```python
from build123d import *

# Parameters (mm, degrees)
F0_W     = 30.6967236102
F0_H     = 108.7295114994
F2_T     = -5
F3_DEPTH = 25
F4_DEPTH = 172.6


with BuildPart() as f1:
    # F0 (on Front) → F1 (revolve)
    with BuildSketch(Plane.XZ):
        with Locations((-15.3483618051, 0)):
            Rectangle(F0_W, F0_H)
    revolve(axis=Axis((0, 0, -2.295082435), (0, 0, -1)))

    # F2
    f2_openings = [f1.faces().sort_by_distance(p)[0] for p in [
        (0, 0, 54.364756),
    ]]
    offset(amount=F2_T, openings=f2_openings)

    # F3 (add): a face of the model
    f3_faces = [f1.faces().sort_by_distance(p)[0] for p in [
        (0, 0, -49.3647557497),
    ]]
    extrude(f3_faces, amount=F3_DEPTH)

    # F4 (add): a face of the model
    f4_faces = [f1.faces().sort_by_distance(p)[0] for p in [
        (0, 0, -24.3647557497),
    ]]
    extrude(f4_faces, amount=F4_DEPTH)


solid = f1.part
```
Geometry: final body of the model. Coordinates: model frame, mm. A direction names the side the tool comes from. Round coordinates to 2 decimals unless told otherwise and drop trailing zeros. Order: outer loops, then holes, each group sorted by start corner. A loop starts at its lowest first (then second) coordinate and runs counter-clockwise, first axis right, second up. Notation, with made-up numbers: (46, 5.25) -> (69, 5.25) arc R13 ccw to (69, 20.25) -> close; hole circle Ø10 at (-31, 0). An arc over 180 degrees is marked (long way). Use one line per item in the form item = value. Start each with the question number.
1. Cut plane A-A (y = 0). Return the cut outline in (x, z), then the cut area to 3 significant figures.
2. Cut plane D-D (z = 119.5). Return the cut outline in (x, y), then the cut area to 3 significant figures.
3. Reachability of faces 1 (the face through (5.571, 25.086, 100.643)), 2 (the face through (0, 0, -54.365)) from +Z, -Z, +X, -X, +Y, -Y: full face, straight path, thin tool, end or side. Return the list, or none.
4. Cut plane B-B (x = 17). Return the cut outline in (y, z).
5. Pin query (flat end, axial travel): pin 1 Ø1.5 at (x, z) = (0, 123.5) entering from +Y; pin 2 Ø8 at (x, z) = (12.5, 106.5) entering from -Y; pin 3 Ø4 at (x, z) = (-1, -18) entering from -Y; pin 4 Ø8 at (y, z) = (2, 2.5) entering from -X. Return the tip coordinate at first contact, or that it passes through.
6. Line query: probe 1 along Z at (x, y) = (-24, 14.5); probe 2 along X at (y, z) = (1.5, 46.5); probe 3 along X at (y, z) = (0, 85). Output: solid intervals per line, ascending.
7. Cut plane C-C (z = 17.5). Return the cut outline in (x, y).
Solution:
q1.outline = (-30.7, -54.36) -> (30.7, -54.36) -> (30.7, 54.36) -> (25.7, 54.36) -> (25.7, 148.24) -> (-25.7, 148.24) -> (-25.7, 54.36) -> (-30.7, 54.36) -> close
q1.area = 11,500 mm^2
q2.outline = circle Ø51.39 at (0, 0)
q2.area = 2,070 mm^2
q3.face_1 = +Z
q3.face_2 = -Z, +X, -X, +Y, -Y
q4.outline = (-25.56, -54.36) -> (25.56, -54.36) -> (25.56, 54.36) -> (19.27, 54.36) -> (19.27, 148.24) -> (-19.27, 148.24) -> (-19.27, 54.36) -> (-25.56, 54.36) -> close
q5.pin_1 = 25.7
q5.pin_2 = -24.25
q5.pin_3 = -30.7
q5.pin_4 = -30.7
q6.probe_1 = -54.36 to 54.36
q6.probe_2 = -30.66 to 30.66
q6.probe_3 = -25.7 to 25.7
q7.outline = circle Ø61.39 at (0, 0)
